Could you check a few things on this model? Use its own coordinates, in mm. Round coordinates to 2 decimals unless told otherwise and drop trailing zeros. Write each loop counter-clockwise with the first axis right and the second up, starting at its lowest first coordinate (ties: lowest second). Pieces come first, ordered by that corner, then holes.
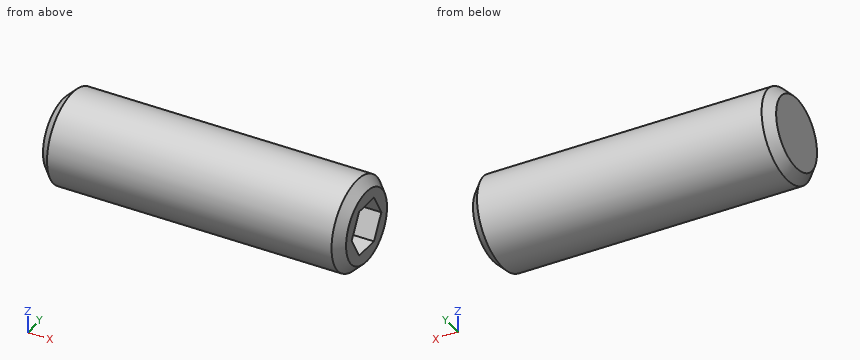
Autodesk Inventor part; units mm, degrees
ref_plane "Work Plane1" through (5, 0, 0) normal (0, 0, 1) x (1, 0, 0)
ref_plane "YZ Plane" through (0, 0, 0) normal (1, 0, 0) x (0, 1, 0)
ref_plane "XZ Plane" through (0, 0, 0) normal (0, 1, 0) x (-1, 0, 0)
sketch "Skizze1" plane through (0, 0, 0) normal (0, 0, 1) x (1, 0, 0)
  line L0 (0, 0) -> (7.5, 0)
  line L1 (10, 0.866) -> (10, 1.5)
  line L2 (10, 1.5) -> (0, 1.5)
  line L3 (10, 0.866) -> (8, 0.866)
  line L4 (8, 0.866) -> (7.5, 0)
  line L5 (0, -0.3) -> (0, 1.8)
  line L6 (0, 1.5) -> (0, 0)
  dimension "d0" = 2
  dimension "d1" = 60
  dimension "d2" = 3
  dimension "d3" = 1.7321
  dimension "d5" = 10
revolve "Körper" add sketch "Skizze1" angle 360 about axis through (0, 0, 0) along (1, 0, 0)
sketch "Skizze2" plane through (10, 0, 0) normal (1, 0, 0) x (0, 1, 0)
  circle A0 centre (0, 0) radius 0.866
  line L0 (-0.433, 0.75) -> (0.433, 0.75)
  line L1 (0.433, 0.75) -> (0.866, 0)
  line L2 (0.866, 0) -> (0.433, -0.75)
  line L3 (0.433, -0.75) -> (-0.433, -0.75)
  line L4 (-0.433, -0.75) -> (-0.866, 0)
  line L5 (-0.866, 0) -> (-0.433, 0.75)
  point P0 (0, 0)
  point P1 (0, 0)
extrude "Loch" add sketch "Skizze2" against normal up to next contours L1 A0 | A0 L2 | L0 A0 | A0 L3 | L5 A0 | A0 L4
thread "Gewinde"
chamfer "Fase1" distance 0.3067 angle 45 1 edges at (10, -1.5, 0) measured on face at (6.6667, 1.4951, -0.1207)
chamfer "Fase2" distance 0.3067 angle 45 1 edges at (0, -1.5, 0) measured on face at (3.2311, 1.4806, -0.2406)
ref_plane "Work Plane1" through (5, 0, 0) normal (0, 0, 1) x (1, 0, 0)
equation "\"d0\" = INTI"
equation "\"d2\" = NND"
equation "\"d3\" = 1.1547 * SW"
equation "\"d5\" = NLG"
equation "\"d8\" = NLG"
equation "\"d10\" = -0.5 * GD1 + 0.5 * NND"
equation "\"d11\" = FAWI"
equation "\"d34\" = -0.5 * GD1 + 0.5 * NND"
equation "\"d12\" = -0.5 * GD1 + 0.5 * NND"
equation "\"d13\" = FAWI"
equation "\"d35\" = -0.5 * GD1 + 0.5 * NND"
equation "\"NND\" = 3"
equation "\"NLG\" = 10"
equation "\"INTI\" = 2"
equation "\"FAWI\" = 45deg"
equation "\"SW\" = 1.5"
equation "\"GD1\" = THREADDIA - 1.2269 * PTC"
equation "\"SPD\" = 2"
equation "\"GUL\" = 0.61345 * PTC"
equation "\"TOA\" = 30deg"
equation "\"THREADDIA\" = 3"
equation "\"PTC\" = 0.5"
equation "\"FAWI1\" = 45deg"
equation "\"GAL\" = 0.61345 * PTC"
equation "\"E0\" = 1.155 * SW"
properties part number "DIN 913 - M3 x 10" material "Stahl, weich"
Q1. Imagine slicing it at B-B, the plane x = 4.5. Write out the boundary of the cut face in (y, z).
Q2. Imagine slicing it at A-A, the plane x = 9.25. Write out the boundary of the cut face in (y, z), then the cut area to 3 significant figures.
Q3. If I drill on L1, parallel to Z at x = 1.75, y = 1.3; L2, parallel to Y at x = 8.5, z = 0.35; L3, parallel to Z at x = 8.75, y = -1.15, over which ranges is the centre line in solid material (lowest first)?
Results found:
1. outline: circle Ø3 at (0, 0)
2. outline: circle Ø3 at (0, 0); hole (-0.87, 0) - (-0.43, -0.75) - (0.43, -0.75) - (0.87, 0) - (0.43, 0.75) - (-0.43, 0.75) - close
2. area: 5.12 mm2
3. L1: z = -0.75 to 0.75
3. L2: y = -1.46 to -0.66, 0.66 to 1.46
3. L3: z = -0.96 to 0.96
